Could you check a few things on this drawing? It's one solid part, dimensions in mm from its lowest x, y, z. A direction names the side the tool comes from. Coordinates: 2 decimals unless noted, no trailing zeros. Order: outer loops, then holes, each group sorted by start corner. A loop starts at its lowest first (then second) coordinate and runs counter-clockwise, first axis right, second up.
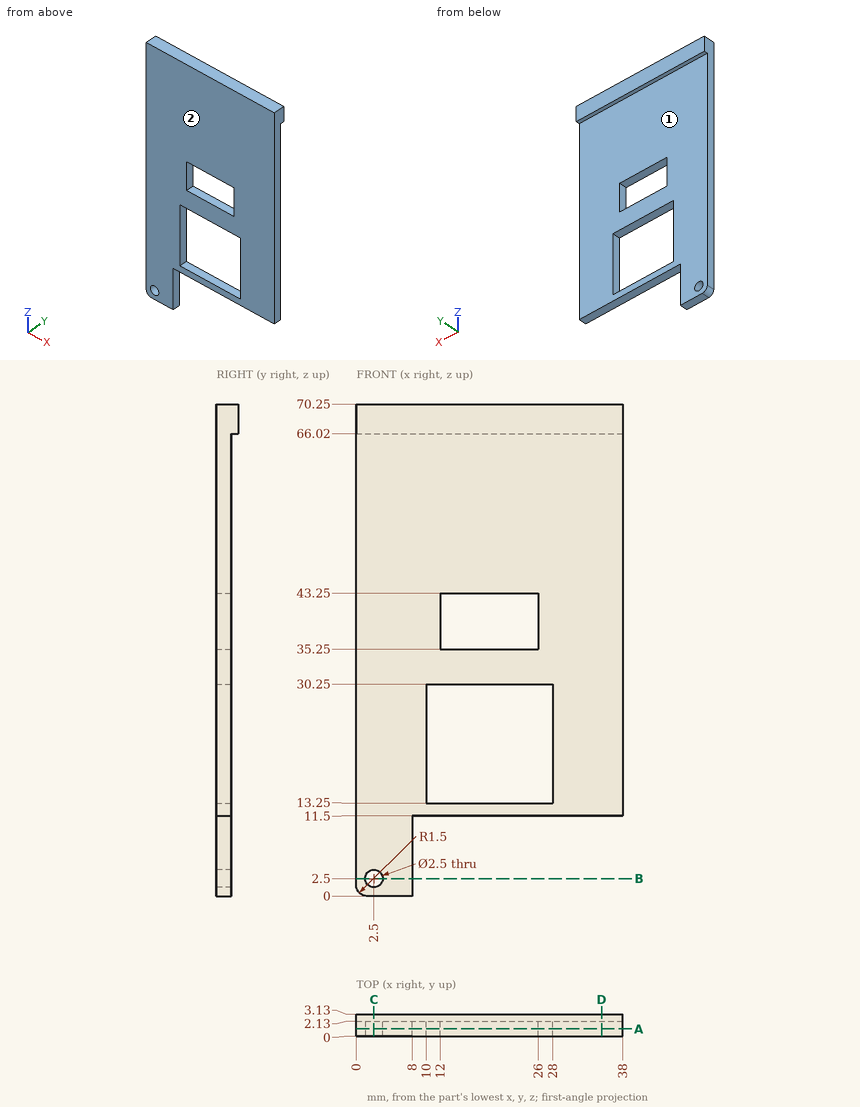
Item 1: Suppose I cut it at B-B (z = 2.5). List the corners of the cut face in (x, y) for me, and give its area (3 significant figures).
Item 2: Suppose I cut it at A-A (y = 1). List the corners of the cut face in (x, z) for me, and give its area (3 significant figures).
Item 3: I need wall thicknesses on line 1 (Z direction, x = 21.5, y = 1.95); line 2 (X direction, y = 1.4, z = 40); line 3 (Z direction, x = 2.5, y = 0.6). Which ranges of each line are inside material? Lowest first, please.
Item 4: For pin 1 Ø0.5 at (x, y) = (18.5, 2.5) entering from -Z; pin 2 Ø1.1 at (y, z) = (1.5, 8.5) entering from +X; pin 3 Ø1.1 at (x, y) = (23, 1) entering from -Z, each with a flat end and sliding along its axis, tell me the tip position at first contact or that it passes through.
Item 5: Which directions (+Z, -Z, +X, -X, +Y, -Y) give clear straight access to the entire face, cutting with the end or side of a thin tool? Please do the marked faces 1 and 2.
Item 6: Suppose I cut it at D-D (x = 35). List the corners of the cut face in (y, z) for me, and give its area (3 significant figures).
Item 7: Suppose I cut it at C-C (x = 2.5). List the corners of the cut face in (y, z) for me, and give its area (3 significant figures).
Geometry results:
1. outline: (0, 0) - (1.25, 0) - (1.25, 2.13) - (0, 2.13) - close; (3.75, 0) - (8, 0) - (8, 2.13) - (3.75, 2.13) - close
1. area: 11.7 mm2
2. outline: (0, 1.5) arc R1.5 ccw to (1.5, 0) - (8, 0) - (8, 11.5) - (38, 11.5) - (38, 70.25) - (0, 70.25) - close; hole circle Ø2.5 at (2.5, 2.5); hole (10, 13.25) - (28, 13.25) - (28, 30.25) - (10, 30.25) - close; hole (12, 35.25) - (26, 35.25) - (26, 43.25) - (12, 43.25) - close
2. area: 1,900 mm2
3. line 1: z = 11.5 to 13.25, 30.25 to 35.25, 43.25 to 70.25
3. line 2: x = 0 to 12, 26 to 38
3. line 3: z = 0 to 1.25, 3.75 to 70.25
4. pin 1: stops at z = 66.02
4. pin 2: stops at x = 8
4. pin 3: stops at z = 11.5
5. face 1: -Z, +X, -X, +Y
5. face 2: +Z, -Z, +X, -X, -Y
6. outline: (0, 11.5) - (2.13, 11.5) - (2.13, 66.02) - (3.13, 66.02) - (3.13, 70.25) - (0, 70.25) - close
6. area: 129 mm2
7. outline: (0, 0) - (2.13, 0) - (2.13, 1.25) - (0, 1.25) - close; (0, 3.75) - (2.13, 3.75) - (2.13, 66.02) - (3.13, 66.02) - (3.13, 70.25) - (0, 70.25) - close
7. area: 149 mm2
